from build123d import *

# Parameters (mm, degrees)
EXTRUDE_1_DEPTH     = 3
SKETCH_3_W          = 20
SKETCH_3_H          = 3
EXTRUDE_2_DEPTH     = 3
FILLET_1_R          = 10
FILLET_2_R          = 3
SKETCH_2_R          = 2
CUT_EXTRUDE_1_DEPTH = 51.490098039
SKETCH_4_R          = 2.5
CUT_EXTRUDE_2_DEPTH = 51.490098039
FILLET_3_R          = 5


with BuildPart() as part:
    # 草图1 → 凸台-拉伸1 (new body)
    with BuildSketch(Plane.XY):
        Polygon((-30, -10), (-30, 10), (-10, 10), (-10, 37.5), (10, 37.5), (10, 10), (30, 10), (30, -10), (10, -10), (10, -37.5), (-10, -37.5), (-10, -10), align=None)
    extrude(amount=EXTRUDE_1_DEPTH)

    # 草图3 → 凸台-拉伸2 (add)
    with BuildSketch(Plane.XY.offset(3)):
        with Locations((0, -39)):
            Rectangle(SKETCH_3_W, SKETCH_3_H)
    extrude(amount=-EXTRUDE_2_DEPTH)

    # 圆角1
    fillet_1_edges = [part.edges().sort_by_distance(p)[0] for p in [
        (-10, 10, 1.5),
        (10, 10, 1.5),
        (-10, -10, 1.5),
    ]]
    fillet(fillet_1_edges, radius=FILLET_1_R)

    # 圆角2
    fillet_2_edges = [part.edges().sort_by_distance(p)[0] for p in [
        (-10, 37.5, 1.5),
        (10, 37.5, 1.5),
        (30, 10, 1.5),
        (30, -10, 1.5),
        (-30, -10, 1.5),
        (-30, 10, 1.5),
        (-10, -40.5, 1.5),
        (10, -40.5, 1.5),
    ]]
    fillet(fillet_2_edges, radius=FILLET_2_R)

    # 草图2 → 切除-拉伸1 (cut, through all)
    with BuildSketch(Plane.XY.offset(3)):
        with Locations((0, 30)):
            Circle(SKETCH_2_R)
        with Locations((0, 15)):
            Circle(SKETCH_2_R)
        with Locations((0, -15)):
            Circle(SKETCH_2_R)
        with Locations((0, -33)):
            Circle(SKETCH_2_R)
    extrude(amount=-CUT_EXTRUDE_1_DEPTH, mode=Mode.SUBTRACT)

    # 草图4 → 切除-拉伸2 (cut, through all)
    with BuildSketch(Plane.XY.offset(3)):
        with Locations((-20, 0)):
            Circle(SKETCH_4_R)
        Circle(SKETCH_4_R)
        with Locations(Location((20, 0, 0), (0, 0, 180))):
            Circle(SKETCH_4_R)
    extrude(amount=-CUT_EXTRUDE_2_DEPTH, mode=Mode.SUBTRACT)

    # 圆角3
    fillet_3_edges = [part.edges().sort_by_distance(p)[0] for p in [
        (10, -10, 1.5),
    ]]
    fillet(fillet_3_edges, radius=FILLET_3_R)


solid = part.part
Input: part model. Units: mm. Frame: model coordinates. A direction names the side the tool comes from. Coordinates: 2 decimals unless noted, no trailing zeros. Write each loop counter-clockwise with the first axis right and the second up, starting at its lowest first coordinate (ties: lowest second). Pieces come first, ordered by that corner, then holes. Notation, with made-up numbers: M -14,-17.75 L 21,-17.75 A25 cw 21,9.25 Z; hole C 53,1.25 d5. An arc over 180 degrees is marked long. Answer as a JSON object with one key per item and string values. Group by question number.
(1) Section B-B on y = 15. Output: boundary loops of the cut face in (x, z).
(2) Contact query for flat-ended pins moving along their axis: P1, Ø0.9, axis at y = -24.5, z = 1, coming from the +X side; P2, Ø1.5, axis at y = 29, z = 1, coming from the -X side; P3, Ø0.9, axis at x = 23.5, z = 1.5, coming from the -Y side. Output: stop coordinate, or through.
(3) Ray query, line 1 along Y through (x, z) = (0, 1.5); line 2 along Y through (x, z) = (-1.5, 2.4); line 3 along Y through (x, z) = (-20, 0.6). Return the intervals inside material, ascending. Write a range as [from, to].
(4) Set-up query: faces 1 (the face through (12, -11, 2)), 2 (the face through (-10, -29, 2)), 3 (the face through (-10, 27, 1)). Return all of +Z, -Z, +X, -X, +Y, -Y with unobstructed straight access to the full face (end or side cutting, diameter ignored); none if empty.
(5) Section D-D on x = -25. Output: boundary loops of the cut face in (y, z).
(6) Mould query, pull axis X, two halves, no side actions, for faces 4 (the face through (0, -13, 2)), 5 (the face through (-22.5, 0.1, 1.5)), 6 (the face through (-30, 0, 1)), 7 (the face through (-7, -1, 3)). Classes: pulls with the +X half, pulls with the -X half, needs draft (parallel to the pull), parting line crosses it, or undercut.
(7) Section A-A on x = 0. Output: boundary loops of the cut face in (y, z).
(8) Section C-C on z = 0.6. Give the number of separate pieces and of enclosed holes in the cut face, plus the area to 3 significant figures.
Result set:
{
 "1": {"outline": "M -11.34,0 L -2,0 L -2,3 L -11.34,3 Z; M 2,0 L 11.34,0 L 11.34,3 L 2,3 Z"},
 "2": {"P1": "stops at x = 10", "P2": "stops at x = -10", "P3": "stops at y = -10"},
 "3": {"line 1": "y = [-40.5, -35], [-31, -17], [-13, -2.5], [2.5, 13], [17, 28], [32, 37.5]", "line 2": "y = [-40.5, -34.32], [-31.68, -16.32], [-13.68, -2], [2, 13.68], [16.32, 28.68], [31.32, 37.5]", "line 3": "y = [-10, -2.5], [2.5, 10]"},
 "4": {"face 1": "+Z, -Z, +X, -Y", "face 2": "+Z, -Z, -X, -Y", "face 3": "+Z, -Z, -X, +Y"},
 "5": {"outline": "M -10,0 L 10,0 L 10,3 L -10,3 Z"},
 "6": {"face 4": "undercut", "face 5": "undercut", "face 6": "pulls with the -X half", "face 7": "needs draft"},
 "7": {"outline": "M -40.5,0 L -35,0 L -35,3 L -40.5,3 Z; M -31,0 L -17,0 L -17,3 L -31,3 Z; M -13,0 L -2.5,0 L -2.5,3 L -13,3 Z; M 2.5,0 L 13,0 L 13,3 L 2.5,3 Z; M 17,0 L 28,0 L 28,3 L 17,3 Z; M 32,0 L 37.5,0 L 37.5,3 L 32,3 Z"},
 "8": {"separate pieces": "1", "enclosed holes": "7", "area": "2,310 mm2"}
}
